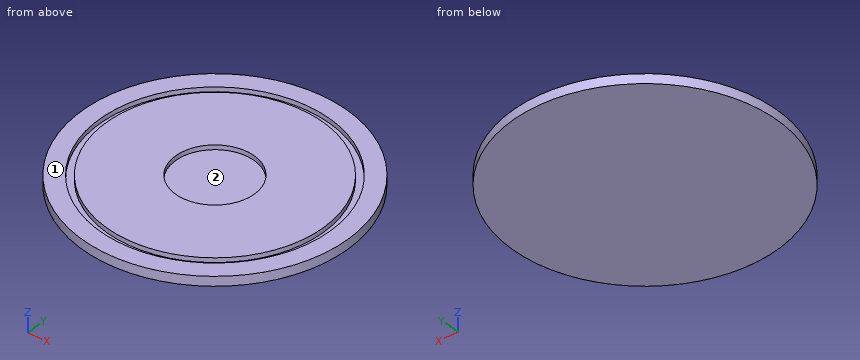
```python
from build123d import *

# Parameters (mm, degrees)
F0_R     = 44.45
F1_DEPTH = 3.175
F2_R     = 38.608
F2_R_2   = 36.322
F2_R_3   = 13.208
F3_DEPTH = 1.524


with BuildPart() as f1:
    # F0 (on Top) → F1 (new body)
    with BuildSketch(Plane.XY):
        Circle(F0_R)
    extrude(amount=F1_DEPTH)

    # F2 (on face) → F3 (cut)
    with BuildSketch(Plane.XY.offset(3.175)):
        Circle(F2_R)
        Circle(F2_R_2, mode=Mode.SUBTRACT)
        Circle(F2_R_3)
    extrude(amount=-F3_DEPTH, mode=Mode.SUBTRACT)


solid = f1.part
```
Here's how the part is built. I have some questions about the finished solid (model axes, mm). Face numbers are marked on the shaded views. Coordinates: 2 decimals unless noted, no trailing zeros. Write each loop counter-clockwise with the first axis right and the second up, starting at its lowest first coordinate (ties: lowest second). Pieces come first, ordered by that corner, then holes. Notation, with made-up numbers: (50.25, 81) -> (104.25, 81) arc R9 ccw to (104.25, 93) -> close; hole circle Ø8 at (-5, -37). An arc over 180 degrees is marked (long way). Use a Markdown table: item, result. Add a question column.
(1) If we section it at D-D, the plane x = 0: Write out the boundary of the cut face in (y, z) (3 decimals), and give its area (3 significant figures).
(2) Please list where these lines run through material, in increasing order: line 1 (Y direction, x = 0, z = 2.45); line 2 (X direction, y = -33.5, z = 2.4); line 3 (Y direction, x = 11.5, z = 1.8).
(3) If we section it at A-A, the plane z = 2.25: Write out the boundary of the cut face in (x, y).
(4) If we section it at B-B, the plane x = -20.5: Write out the boundary of the cut face in (y, z) (1 decimal), and give its area (3 significant figures).
(5) If we section it at C-C, the plane y = 5: Write out the boundary of the cut face in (x, z) (3 decimals).
(6) I'm going to push flat-ended pins straight in: P1, Ø1.5, axis at x = -2.5, z = 1, coming from the +Y side; P2, Ø1.5, axis at x = -26.5, z = 1.5, coming from the -Y side; P3, Ø24, axis at x = 0, y = 0, coming from the +Z side. Where does each tip first touch, or does it pass through?
(7) We'd pull the mould along X, two halves only. Please class the marked faces 1 and 2: +X half, -X half, draft (parallel to the pull), parting line (faces both ways), or undercut.
Outcome:
| question | item | result |
|---|---|---|
| 1 | outline | (-44.45, 0) -> (44.45, 0) -> (44.45, 3.175) -> (38.608, 3.175) -> (38.608, 1.651) -> (36.322, 1.651) -> (36.322, 3.175) -> (13.208, 3.175) -> (13.208, 1.651) -> (-13.208, 1.651) -> (-13.208, 3.175) -> (-36.322, 3.175) -> (-36.322, 1.651) -> (-38.608, 1.651) -> (-38.608, 3.175) -> (-44.45, 3.175) -> close |
| 1 | area | 235 mm^2 |
| 2 | line 1 | y = -44.45 to -38.61, -36.32 to -13.21, 13.21 to 36.32, 38.61 to 44.45 |
| 2 | line 2 | x = -29.22 to -19.19, -14.04 to 14.04, 19.19 to 29.22 |
| 2 | line 3 | y = -42.94 to -36.86, -34.45 to -6.5, 6.5 to 34.45, 36.86 to 42.94 |
| 3 | outline | circle Ø88.9 at (0, 0); circle Ø72.64 at (0, 0); hole circle Ø77.22 at (0, 0); hole circle Ø26.42 at (0, 0) |
| 4 | outline | (-39.4, 0) -> (39.4, 0) -> (39.4, 3.2) -> (32.7, 3.2) -> (32.7, 1.7) -> (30, 1.7) -> (30, 3.2) -> (-30, 3.2) -> (-30, 1.7) -> (-32.7, 1.7) -> (-32.7, 3.2) -> (-39.4, 3.2) -> close |
| 4 | area | 242 mm^2 |
| 5 | outline | (-44.168, 0) -> (44.168, 0) -> (44.168, 3.175) -> (38.283, 3.175) -> (38.283, 1.651) -> (35.976, 1.651) -> (35.976, 3.175) -> (12.225, 3.175) -> (12.225, 1.651) -> (-12.225, 1.651) -> (-12.225, 3.175) -> (-35.976, 3.175) -> (-35.976, 1.651) -> (-38.283, 1.651) -> (-38.283, 3.175) -> (-44.168, 3.175) -> close |
| 6 | P1 | stops at y = 44.42 |
| 6 | P2 | stops at y = -36.23 |
| 6 | P3 | stops at z = 1.65 |
| 7 | face 1 | draft |
| 7 | face 2 | undercut |
